Here's how the part is built. I have some questions about the finished solid (model axes, mm). Coordinates: 2 decimals unless noted, no trailing zeros. Loops run counter-clockwise (first coordinate to the right, second up) from the corner with the lowest first, then second, coordinate; pieces in that order, holes last. Notation, with made-up numbers: (43, 71) -> (72, 71) arc R22 ccw to (72, 89) -> close; hole circle Ø9 at (-33.5, -22). An arc over 180 degrees is marked (long way). Answer as a JSON object with one key per item and string values. Group by question number.
Q1. I'm going to push flat-ended pins straight in: pin 1 (1.5 mm diameter, centred on x = 27, z = 1.5, fed in from -Y); pin 2 (1.5 mm diameter, centred on x = 27.5, z = 2, fed in from +Y); pin 3 (0.9 mm diameter, centred on y = 31, z = 2.5, fed in from +X) (3 decimals). Where does each tip first touch, or does it pass through?
Q2. I want a section at C-C on y = 4. Write out the boundary of the cut face in (x, z) (3 decimals).
Q3. I need wall thicknesses on line 1 (Y direction, x = -22.5, z = 0.7); line 2 (Y direction, x = 27, z = 1.9); line 3 (Y direction, x = -9, z = 2) (3 decimals). Which ranges of each line are inside material? Lowest first, please.
Q4. I want a section at A-A on z = 2.35. Write out the boundary of the cut face in (x, y) (3 decimals).
Q5. I want a section at B-B on x = -3.5. Write out the boundary of the cut face in (y, z) (3 decimals), then the cut area to 3 significant figures.
```python
from build123d import *

# Parameters (mm, degrees)
F0_W     = 58
F0_H     = 63.5
F1_DEPTH = 3.175
F2_W     = 37.8
F2_H     = 3.075
F2_W_2   = 3.075
F2_H_2   = 14.3
F2_H_3   = 9.9
F3_DEPTH = 25
F5_DEPTH = 25


# Not quite as in the source:
# - a length typed as a fraction of an inch, garbled in the dataset ("3 / 203.2 mm" for 3/8 in), is restored


with BuildPart() as f1:
    # F0 (on Top) → F1 (new body)
    with BuildSketch(Plane.XY):
        Rectangle(F0_W, F0_H)
    extrude(amount=F1_DEPTH)

    # F2 (on face) → F3 (cut)
    with BuildSketch(Plane.XY.offset(3.175)):
        with Locations((0, -30.2125)):
            Rectangle(F2_W, F2_H)
        with Locations((0, 30.2125)):
            Rectangle(F2_W, F2_H)
        with Locations((27.4625, 0)):
            Rectangle(F2_W_2, F2_H_2)
        with Locations((27.4625, -26.8)):
            Rectangle(F2_W_2, F2_H_3)
        with Locations((27.4625, 26.8)):
            Rectangle(F2_W_2, F2_H_3)
    extrude(amount=-F3_DEPTH, mode=Mode.SUBTRACT)

    # F4 (on face) → F5 (cut)
    with BuildSketch(Plane.XY.offset(3.175)):
        with BuildLine():
            ThreePointArc((-15.6, -24.08), (-20.68, -19), (-15.6, -13.92))
            Line((-15.6, -13.92), (-29, -13.92))
            Line((-29, -13.92), (-29, -24.08))
            Line((-29, -24.08), (-15.6, -24.08))
        make_face()
        with BuildLine():
            ThreePointArc((-15.6, -24.08), (-12.0078975516, -22.5921024484), (-10.52, -19))
            ThreePointArc((-10.52, -19), (-12.0078975516, -15.4078975516), (-15.6, -13.92))
            ThreePointArc((-15.6, -13.92), (-20.68, -19), (-15.6, -24.08))
        make_face()
    extrude(amount=-F5_DEPTH, mode=Mode.SUBTRACT)


solid = f1.part
```
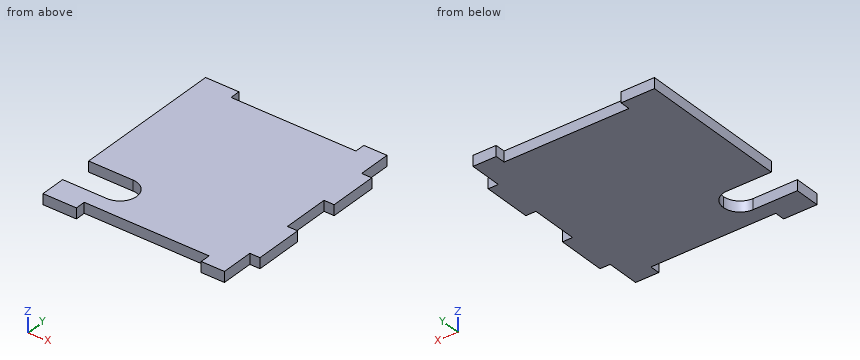
Result set:
{
 "1": {"pin 1": "stops at y = -21.85", "pin 2": "stops at y = 21.85", "pin 3": "stops at x = 25.925"},
 "2": {"outline": "(-29, 0) -> (25.925, 0) -> (25.925, 3.175) -> (-29, 3.175) -> close"},
 "3": {"line 1": "y = -31.75 to -24.08, -13.92 to 31.75", "line 2": "y = -21.85 to -7.15, 7.15 to 21.85", "line 3": "y = -28.675 to 28.675"},
 "4": {"outline": "(-29, -31.75) -> (-18.9, -31.75) -> (-18.9, -28.675) -> (18.9, -28.675) -> (18.9, -31.75) -> (25.925, -31.75) -> (25.925, -21.85) -> (29, -21.85) -> (29, -7.15) -> (25.925, -7.15) -> (25.925, 7.15) -> (29, 7.15) -> (29, 21.85) -> (25.925, 21.85) -> (25.925, 31.75) -> (18.9, 31.75) -> (18.9, 28.675) -> (-18.9, 28.675) -> (-18.9, 31.75) -> (-29, 31.75) -> (-29, -13.92) -> (-15.6, -13.92) arc R5.08 cw to (-15.6, -24.08) -> (-29, -24.08) -> close"},
 "5": {"outline": "(-28.675, 0) -> (28.675, 0) -> (28.675, 3.175) -> (-28.675, 3.175) -> close", "area": "182 mm²"}
}
